Design review of the part built by this model. Coordinates are the model's own, in mm. A direction names the side the tool comes from. Give positions to 0.01 mm unless a question says otherwise; leave off trailing zeros. Write each loop counter-clockwise with the first axis right and the second up, starting at its lowest first coordinate (ties: lowest second). Pieces come first, ordered by that corner, then holes. Notation, with made-up numbers: (2.5, 62) -> (23.5, 62) arc R10 cw to (23.5, 69) -> close; hole circle Ø8 at (80.5, -32). An arc over 180 degrees is marked (long way). Use CSV: the item, a comma, the result in double quotes.
Autodesk Inventor part; units mm, degrees
ref_plane "YZ Plane" through (0, 0, 0) normal (1, 0, 0) x (0, 1, 0)
ref_plane "XZ Plane" through (0, 0, 0) normal (0, 1, 0) x (-1, 0, 0)
ref_plane "XY Plane" through (0, 0, 0) normal (0, 0, 1) x (1, 0, 0)
sketch "Sketch1" plane through (0, 0, 0) normal (0, 1, 0) x (-1, 0, 0)
  circle A0 centre (0, 0) radius 2.1
  circle A1 centre (0, 0) radius 8
  circle A2 centre (0, 0) radius 12.5
  circle A3 centre (0, 0) radius 51.9615
  line L0 (-45, -25.9808) -> (-28.034, 3.4052)
  line L1 (0, 51.9615) -> (16.966, 22.5755)
  line L2 (45, -25.9808) -> (11.068, -25.9808)
  circle A4 centre (12.5, 30.3109) radius 5
  circle A5 centre (32.5, -4.3301) radius 5
  circle A6 centre (-12.5, 30.3109) radius 5
  circle A7 centre (-32.5, -4.3301) radius 5
  circle A8 centre (-20, -25.9808) radius 5
  circle A9 centre (20, -25.9808) radius 5
  circle A10 centre (0, 12.5) radius 1.6
  circle A11 centre (-10.8253, 6.25) radius 1.6
  circle A12 centre (-10.8253, -6.25) radius 1.6
  circle A13 centre (0, -12.5) radius 1.6
  circle A14 centre (10.8253, -6.25) radius 1.6
  circle A15 centre (10.8253, 6.25) radius 1.6
  circle A16 centre (-32.5, -4.3301) radius 7.5
  circle A17 centre (-12.5, 30.3109) radius 7.5
  circle A18 centre (12.5, 30.3109) radius 7.5
  circle A19 centre (32.5, -4.3301) radius 7.5
  circle A20 centre (20, -25.9808) radius 7.5
  circle A21 centre (-20, -25.9808) radius 7.5
  arc A22 (-8.75, 36.8061) -> (8.75, 36.8061) centre (0, 51.9615) ccw
  arc A23 (-27.5, -25.9808) -> (-36.25, -10.8253) centre (-45, -25.9808) ccw
  arc A24 (36.25, -10.8253) -> (27.5, -25.9808) centre (45, -25.9808) ccw
  arc A25 (13.2584, -29.2673) -> (-13.2584, -29.2673) centre (0, -35.7308) ccw
  arc A26 (-31.9754, 3.1515) -> (-18.717, 26.1158) centre (-30.9437, 17.8654) ccw
  arc A27 (18.717, 26.1158) -> (31.9754, 3.1515) centre (30.9437, 17.8654) ccw
  line L3 (-16.966, 22.5755) -> (0, 51.9615)
  line L4 (-28.034, 3.4052) -> (-16.966, 22.5755)
  line L5 (-11.068, -25.9808) -> (-45, -25.9808)
  line L6 (11.068, -25.9808) -> (-11.068, -25.9808)
  line L7 (16.966, 22.5755) -> (28.034, 3.4052)
  line L8 (28.034, 3.4052) -> (45, -25.9808)
  circle A28 centre (14.0253, 0) radius 1.6
  point P0 (-28.75, 2.1651)
  point P1 (-16.25, 23.8157)
  point P2 (16.25, 23.8157)
  point P3 (28.75, 2.1651)
  point P4 (12.5, -25.9808)
  point P5 (-12.5, -25.9808)
  dimension "d4" = 25
  dimension "d0" = 4.2
  dimension "d3" = 16
  dimension "d11" = 90
  dimension "d12" = 40
  dimension "d13" = 10
  dimension "d14" = 25
  dimension "d15" = 25
  dimension "d16" = 40
  dimension "d17" = 40
  dimension "d18" = 25
  dimension "d19" = 25
  dimension "d26" = 3.2
  dimension "d29" = 360
  dimension "d38" = 15
  dimension "d47" = 5
  dimension "d48" = 90
  dimension "d49" = 90
  dimension "d50" = 6.25
  dimension "d51" = 3.2
extrude "Shape" add sketch "Sketch1" along normal blind 6.731 contours A1 | A2 A28 | A2 A28 | A28 A2 A14 A13 A12 A11 A10 A15 | A15 A2 | A2 A15 | A14 A2 | A2 A14 | A10 A2 | A2 A10 | A13 A2 | A2 A13 | A11 A2 | A2 A11 | A12 A2 | A2 A12 | A18 L1 A4 | L1 A4 A18 | A18 L1 A27 L8 A19 A24 A20 L2 A25 L5 A21 A23 A16 L0 A26 L3 A17 A22 | L3 A6 A17 | A17 L3 A6 | A20 L2 A9 | L2 A9 A20 | L8 A5 A19 | A19 L8 A5 | A16 L0 A7 | L0 A7 A16 | L5 A8 A21 | A21 L5 A8 | A4 L1 | L1 A4 | A18 A27 L1 | A17 L3 A26 | L3 A6 | A6 L3 | A9 L2 | L2 A9 | A25 L2 A20 | L8 A27 A19 | L8 A5 | A5 L8 | A7 L0 | L0 A7 | A26 L0 A16 | L5 A25 A21 | L5 A8 | A8 L5
extrude "Holes" cut sketch "Sketch1" along normal up to next contours A2 A28 | A2 A28 | A15 A2 | A2 A15 | A14 A2 | A2 A14 | A10 A2 | A2 A10 | A13 A2 | A2 A13 | A11 A2 | A2 A11 | A12 A2 | A2 A12 | A4 L1 | L1 A4 | L3 A6 | A6 L3 | A9 L2 | L2 A9 | L8 A5 | A5 L8 | A7 L0 | L0 A7 | L5 A8 | A8 L5
extrude "Inset" cut sketch "Sketch1" along normal blind 3.231 contours A1
sketch "Sketch2" plane through (0, 6.731, 0) normal (0, 1, 0) x (1, 0, 0)
  circle A0 centre (-14.0253, 0) radius 1.6
extrude "Extrusion7" add sketch "Sketch2" against normal up to surface (6.731 mm away)
equation "\"d14\" = d15"
equation "\"d16\" = d12"
equation "\"d17\" = d12"
equation "\"d18\" = d14"
equation "\"d19\" = d14"
equation "\"d48\" = d11"
equation "\"d49\" = d11"
equation "\"d43\" = THICKB"
equation "\"THICKA\" = 3.175"
equation "\"THICKB\" = 6.731"
equation "\"THICKC\" = 12.7"
equation "\"MAGDIA\" = 9.5"
equation "\"BALLDIA\" = 12"
properties part number "Effector_Platform"
(1) Tool access review of faces 1 (the face through (-17.888, 3.318, 35.528)), 2 (the face through (-2, 3.231, -2)): name each direction out of +Z, -Z, +X, -X, +Y, -Y from which nothing blocks a thin tool from reaching the whole face with its end or side.
Established:
face 1,"+Y, -Y"
face 2,"-Y"
(2) Mouldability with a two-part tool opening along Z and no side actions: class faces 3 (the face through (-8, 0, 3)), 4 (the face through (-0.128, 3.318, 34.462)), 5 (the face through (-15, 3, -26)) as +Z half, -Z half, draft (parallel to the pull), parting line (faces both ways), or undercut.
Established:
face 3,"draft"
face 4,"+Z half"
face 5,"undercut"
(3) Clearance check with flat-ended pins moving along their axes: pin 1 (1 mm diameter, centred on x = -10.5, y = 3.5, fed in from +Z); pin 2 (1.9 mm diameter, centred on x = 10.83, z = -6.25, fed in from -Y); pin 3 (1 mm diameter, centred on y = 5.5, z = 26.5, fed in from -X); pin 4 (1 mm diameter, centred on y = 5, z = 27, fed in from +X). State where each tip first meets the part, or that it passes through.
Established:
pin 1,"stops at z = 37.66"
pin 2,"passes through"
pin 3,"stops at x = -19.23"
pin 4,"stops at x = 19.45"
(4) Take a section at A-A (x = -11). Write out the cut boundary in (y, z), then the cut area to 3 significant figures.
Established:
outline,"(0, -25.9) -> (6.73, -25.9) -> (6.73, -7.84) -> (0, -7.84) -> close; (0, -4.66) -> (6.73, -4.66) -> (6.73, 4.66) -> (0, 4.66) -> close; (0, 7.84) -> (6.73, 7.84) -> (6.73, 25.54) -> (0, 25.54) -> close; (0, 35.08) -> (6.73, 35.08) -> (6.73, 37.66) -> (0, 37.66) -> close"
area,"321 mm2"
(5) For line 1 along Z through (x, y) = (0, 1.1); line 2 along X through (y, z) = (5.5, 34); line 3 along X through (y, z) = (4, 6.25), list the stretches that pass through material, from the lowest coordinate up. Write a range as [from, to].
Established:
line 1,"z = [-20.98, -14.1], [-10.9, -8], [8, 10.9], [14.1, 34.46]"
line 2,"x = [-19.03, -15.87], [-9.13, 9.13], [15.87, 19.03]"
line 3,"x = [-21.85, -12.43], [-9.23, 9.23], [12.43, 21.85]"
(6) Take a section at D-D (z = 12.5). Write out the cut boundary in (x, y).
Established:
outline,"(-17.2, 0) -> (-1.6, 0) -> (-1.6, 6.73) -> (-17.2, 6.73) -> close; (1.6, 0) -> (17.2, 0) -> (17.2, 6.73) -> (1.6, 6.73) -> close"
(7) Take a section at B-B (z = -6.25). Write out the cut boundary in (x, y).
Established:
outline,"(-39.75, 0) -> (-37.12, 0) -> (-37.12, 6.73) -> (-39.75, 6.73) -> close; (-27.88, 0) -> (-12.43, 0) -> (-12.43, 6.73) -> (-27.88, 6.73) -> close; (-9.23, 0) -> (-4.99, 0) -> (-4.99, 3.23) -> (4.99, 3.23) -> (4.99, 0) -> (9.23, 0) -> (9.23, 6.73) -> (-9.23, 6.73) -> close; (12.43, 0) -> (27.88, 0) -> (27.88, 6.73) -> (12.43, 6.73) -> close; (37.12, 0) -> (39.75, 0) -> (39.75, 6.73) -> (37.12, 6.73) -> close"
(8) Take a section at C-C (x = -35). Write out the cut boundary in (y, z).
Established:
outline,"(0, -11.62) -> (6.73, -11.62) -> (6.73, -8.66) -> (0, -8.66) -> close; (0, 0) -> (6.73, 0) -> (6.73, 2.74) -> (0, 2.74) -> close"
